Model file for the job. Use its own axes, mm. A direction names the side the tool comes from. Round coordinates to 2 decimals unless told otherwise and drop trailing zeros. Order: outer loops, then holes, each group sorted by start corner. A loop starts at its lowest first (then second) coordinate and runs counter-clockwise, first axis right, second up. Notation, with made-up numbers: (0, -36) -> (15, -36) arc R26 ccw to (15, -2) -> close; hole circle Ø1 at (7, 30). An arc over 180 degrees is marked (long way). Use CSV: the item, a comma, the result in double quotes.
```python
from build123d import *

# Parameters (mm, degrees)
CUT_EXTRUDE1_DEPTH = 0.25


with BuildPart() as part:
    # Sketch1 → Revolve1 (revolve)
    with BuildSketch(Plane(origin=(0, 0, 0), x_dir=(0, 0, -1), z_dir=(1, 0, 0)), mode=Mode.PRIVATE) as revolve1_sk:
        Polygon((0, 0), (0, 3), (2.4, 3), (2.4, 1.5), (5.4, 1.5), (5.4, 0), align=None)
    revolve(revolve1_sk.sketch.rotate(Axis((0, 0, 0), (0, 0, -1)), 90), axis=Axis((0, 0, 0), (0, 0, -1)))

    # Sketch2 → Cut-Extrude1 (cut)
    with BuildSketch(Plane.XY):
        Polygon((-0.25, 3), (-0.25, 0.25), (-3, 0.25), (-3.446498645, 0), (-3, -0.25), (-0.25, -0.25), (-0.25, -2), (-0.25, -3.474150095), (0.25, -3.474150095), (0.25, -2), (0.25, -0.25), (2, -0.25), (3.076862429, -0.25), (4.006902363, -0.319251284), (4.006902363, 0.25), (2, 0.25), (0.25, 0.25), (0.25, 3), (0, 3.446498645), align=None)
    extrude(amount=-CUT_EXTRUDE1_DEPTH, mode=Mode.SUBTRACT)


solid = part.part
```
Q1. Probe line 1 along Z through (x, y) = (1.3, -2.6); line 2 along Z through (x, y) = (1.6, -0.1); line 3 along X through (y, z) = (0.6, -0.2). List the from-to ranges inside material, lowest first.
From the geometry:
line 1,"z = -2.4 to 0"
line 2,"z = -2.4 to -0.25"
line 3,"x = -2.94 to -0.25, 0.25 to 2.94"
Q2. Which spindle directions (+Z, -Z, +X, -X, +Y, -Y) get a long thin tool onto all of the face, cutting with end or side? Do faces 1 (the cylindrical face through (1.43, -0.45, -3.92)), 2 (the flat face through (1, -1, 0)). Say none if no direction does.
From the geometry:
face 1,"-Z"
face 2,"+Z, +X, -X, +Y, -Y"
Q3. Pin check, flat tips, straight feed: pin 1 (1.5 mm diameter, centred on x = 2, z = -1.5, fed in from +Y); pin 2 (1 mm diameter, centred on y = 2, z = -1, fed in from -X); pin 3 (1 mm diameter, centred on x = -2, z = -2, fed in from +Y). Stop position of each tip, or through.
From the geometry:
pin 1,"stops at y = 2.73"
pin 2,"stops at x = -2.6"
pin 3,"stops at y = 2.6"
Q4. Cut at A-A (y = 0). Give the cut face in (x, z).
From the geometry:
outline,"(-3, -2.4) -> (-1.5, -2.4) -> (-1.5, -5.4) -> (1.5, -5.4) -> (1.5, -2.4) -> (3, -2.4) -> (3, -0.25) -> (-3, -0.25) -> close"
Q5. Cut at D-D (y = 0.75). Give the cut face in (x, z).
From the geometry:
outline,"(-2.9, -2.4) -> (-1.3, -2.4) -> (-1.3, -5.4) -> (1.3, -5.4) -> (1.3, -2.4) -> (2.9, -2.4) -> (2.9, 0) -> (0.25, 0) -> (0.25, -0.25) -> (-0.25, -0.25) -> (-0.25, 0) -> (-2.9, 0) -> close"
Q6. Cut at C-C (z = -1.25). Give the cut face in (x, y), plus the area to 3 significant figures.
From the geometry:
outline,"circle Ø6 at (0, 0)"
area,"28.3 mm²"
Q7. Mould opens along Y. For faces 3 (the flat face through (-1, -1, 0)), 4 (the flat face through (0, 0, -0.25)), 5 (the cylindrical face through (2.86, -0.9, -1.22)) say: +Y half, -Y half, draft (parallel to the pull), parting line (faces both ways), or undercut.
From the geometry:
face 3,"draft"
face 4,"undercut"
face 5,"parting line"
